Build history of the part. All positions in model axes, mm. A direction names the side the tool comes from. Round coordinates to 2 decimals unless told otherwise and drop trailing zeros. Order: outer loops, then holes, each group sorted by start corner. A loop starts at its lowest first (then second) coordinate and runs counter-clockwise, first axis right, second up. Notation, with made-up numbers: M -3,-29.5 L 32,-29.5 A21 ccw 32,-7.5 Z; hole C 10.5,23 d1. An arc over 180 degrees is marked long. One line per question, with ' | ' between items. Start each with the question number.
Autodesk Inventor part; units mm, degrees
ref_plane "YZ Plane" through (0, 0, 0) normal (1, 0, 0) x (0, 1, 0)
ref_plane "XZ Plane" through (0, 0, 0) normal (0, 1, 0) x (-1, 0, 0)
ref_plane "XY Plane" through (0, 0, 0) normal (0, 0, 1) x (1, 0, 0)
sketch "Sketch1" plane through (0, 0, 0) normal (0, 0, 1) x (1, 0, 0)
  line L0 (0, 0) -> (0, 81.958)
  line L1 (0, 0) -> (0, -81.958)
  line L2 (0, -81.958) -> (-10, -81.958)
  line L3 (-5, -81.958) -> (-5, -67.708) construction
  line L4 (-5, -67.708) -> (-5, -58.708) construction
  line L5 (-10, -81.958) -> (-10, -58.708)
  line L6 (-10, -58.708) -> (0, -58.708)
  line L7 (0, 81.958) -> (-10, 81.958)
  line L8 (-5, 81.958) -> (-5, 66.21) construction
  line L9 (-5, 66.21) -> (-5, 20.031) construction
  line L10 (-5, 20.031) -> (-5, 11.031) construction
  line L11 (-10, 81.958) -> (-10, 11.031)
  line L12 (-10, 11.031) -> (0, 11.031)
  line L13 (0, -58.708) -> (-2, -58.708)
  line L14 (-2, -58.708) -> (-2, 11.031)
  line L15 (0, -81.958) -> (8, -81.958)
  line L16 (8, -81.958) -> (8, 81.958)
  line L17 (8, 81.958) -> (0, 81.958)
  line L18 (0, 81.958) -> (0, -81.958)
  dimension "d0" = 81.958
  dimension "d2" = 163.916
  dimension "d3" = 10
  dimension "d4" = 14.25
  dimension "d5" = 9
  dimension "d6" = 15.748
  dimension "d7" = 46.179
  dimension "d8" = 9
  dimension "d9" = 2
  dimension "d10" = 8
extrude "Extrusion1" add sketch "Sketch1" along normal blind 7
sketch "Sketch2" plane through (0, 0, 0) normal (0, 0, -1) x (-1, 0, 0)
  line L0 (10, 81.958) -> (10, 11.031) construction
  line L1 (10, 46.4945) -> (-5, 46.4945) construction
  line L2 (-50, 81.958) -> (-50, -81.958)
  line L3 (-35.1508, -57.5) -> (-20.1508, -57.5)
  line L4 (-20.1508, -57.5) -> (-20.1508, 57.5)
  line L5 (-20.1508, 57.5) -> (-35.1508, 57.5)
  line L6 (-35.1508, 57.5) -> (-35.1508, -57.5)
  line L7 (-35.1508, -57.5) -> (-20.1508, 57.5) construction
  line L8 (-20.1508, -57.5) -> (-35.1508, 57.5) construction
  line L9 (-5, -81.958) -> (-5, 81.958)
  line L10 (-50, -81.958) -> (-5, -81.958)
  line L11 (10, -81.958) -> (-8, -81.958)
  line L12 (-50, 81.958) -> (-5, 81.958)
  line L13 (-8, 81.958) -> (10, 81.958)
  point P0 (0, 0)
  point P1 (-27.6508, 0)
  dimension "d13" = 15
  dimension "d15" = 15
  dimension "d16" = 115
extrude "Extrusion2" add sketch "Sketch2" along normal blind 9
sketch "Sketch3" plane through (-10, -81.958, 7) normal (0, -1, 0) x (1, 0, 0)
  line L0 (18, -7) -> (60, -7)
  line L1 (60, -7) -> (18, -7)
  line L2 (18, -7) -> (18, -2)
  line L3 (18, -7) -> (18, 0)
  line L4 (18, -2) -> (60, -2)
  line L5 (60, -2) -> (60, -7)
  line L6 (18, -2) -> (30, -2) construction
  line L7 (60, -2) -> (48, -2) construction
  arc A0 (30, -2) -> (48, -2) centre (39, 20.1797) ccw
  dimension "d34" = 5
  dimension "d35" = 12
  dimension "d36" = 12
extrude "Extrusion3" add sketch "Sketch3" against normal up to surface (24.458 mm away) contours L2 L4 A0 L5 L0
mirror "Mirror1" about plane through (0, 0, 0) normal (0, 1, 0) of "Extrusion3"
sketch "Sketch4" plane through (0, 0, 7) normal (0, 0, 1) x (1, 0, 0)
  line L0 (-5, -81.958) -> (-5, -67.708) construction
  line L1 (-5, 81.958) -> (-5, 66.21) construction
  line L2 (-5, 66.21) -> (-5, 20.031) construction
  line L3 (-10, -58.708) -> (-10, -81.958) construction
  line L4 (-10, -70.333) -> (5, -70.333) construction
  line L5 (5, 81.958) -> (5, -81.958) construction
  circle A0 centre (-2.5, -67.708) radius 1.65
  circle A1 centre (-2.5, 20.031) radius 1.65
  circle A2 centre (-2.5, 66.21) radius 1.65
  point P0 (0, 0)
  dimension "d22" = 14.25
  dimension "d23" = 46.179
  dimension "d24" = 15.748
  dimension "d31" = 15
  dimension "d32" = 3.3
extrude "Extrusion4" cut sketch "Sketch4" against normal up to surface (7 mm away)
sketch "Sketch5" plane through (0, 0, 7) normal (0, 0, 1) x (1, 0, 0)
  circle A0 centre (-2.5, -67.708) radius 1.65
  circle A1 centre (-2.5, -67.708) radius 2.65
  circle A2 centre (-2.5, 20.031) radius 1.65
  circle A3 centre (-2.5, 20.031) radius 2.65
  circle A4 centre (-2.5, 66.21) radius 1.65
  circle A5 centre (-2.5, 66.21) radius 2.65
  dimension "d33" = 5.3
extrude "Extrusion5" cut sketch "Sketch5" against normal blind 6 contours A0 | A1 | A2 | A3 | A4 | A5
fillet "Fillet1" radius 4 2 edges at (50, -81.958, -2) (50, 81.958, -2)
fillet "Fillet2" radius 2 2 edges at (8, -69.729, 5) (8, 69.729, 5)
properties part number "Base Extension 2"
Item 1: Cut at A-A on x = 29. Write the cut outline in (y, z), then the cut area to 3 significant figures.
Item 2: Cut at D-D on y = 15. Write the cut outline in (x, z), then the cut area to 3 significant figures.
Item 3: Two-plate mould, pull along Y, no slides. Class faces 4 (the face through (5, -1, -4)), 5 (the face through (29, -57.5, -1)), 6 (the face through (48.797, 80.817, -2.098)): +Y half, -Y half, draft (parallel to the pull), parting line (faces both ways), or undercut.
Item 4: Tool access for faces 1 (the face through (14, 1, 0)), 2 (the face through (15, -70, 5)), 3 (the face through (20.151, -1, -4)): list every direction of +Z, -Z, +X, -X, +Y, -Y with a clear straight run to the whole face (end or side of a thin tool).
Item 5: Cut at B-B on z = -5.25. Write the cut outline in (x, y).
Item 6: Wall check: line 1 along Y through (x, z) = (-2.5, 2.4); line 2 along Y through (x, z) = (-2.5, 0.75); line 3 along Y through (x, z) = (28, 2). Give the ranges that are in metal, low to high. Write a range as [from, to].
Item 7: Flat gauge pins, fed straight in: pin 1 (3.5 mm diameter, centred on y = -12.5, z = 2.5, fed in from +X); pin 2 (4.5 mm diameter, centred on x = -2.5, y = 66.21, fed in from -Z); pin 3 (10 mm diameter, centred on x = 39, y = -54, fed in from +Z). Where does each tip first touch, or does it go through?
Results found:
1) outline: M -81.96,-9 L -57.5,-9 L -57.5,3.24 L -81.96,3.24 Z; M 57.5,-9 L 81.96,-9 L 81.96,3.24 L 57.5,3.24 Z | area: 599 mm^2
2) outline: M -10,0 L 5,0 L 5,-9 L 20.15,-9 L 20.15,0 L 8,0 L 8,7 L -10,7 Z; M 35.15,-9 L 50,-9 L 50,0 L 35.15,0 Z | area: 396 mm^2
3) face 4: draft | face 5: undercut | face 6: +Y half
4) face 1: +Z, +X | face 2: +Z, +X, +Y, -Y | face 3: +Z, -Z
5) outline: M 5,-81.96 L 46,-81.96 A4 ccw 50,-77.96 L 50,77.96 A4 ccw 46,81.96 L 5,81.96 Z; hole M 20.15,-57.5 L 35.15,-57.5 L 35.15,57.5 L 20.15,57.5 Z
6) line 1: y = [-81.96, -70.36], [-65.06, -58.71], [11.03, 17.38], [22.68, 63.56], [68.86, 81.96] | line 2: y = [-81.96, -69.36], [-66.06, -58.71], [11.03, 18.38], [21.68, 64.56], [67.86, 81.96] | line 3: y = [-81.96, -57.5], [57.5, 81.96]
7) pin 1: stops at x = 8 | pin 2: stops at z = 0 | pin 3: stops at z = 5
